Here's how the part is built. I have some questions about the finished solid (model axes, mm). Face numbers are marked on the shaded views. A direction names the side the tool comes from. Give positions to 0.01 mm unless a question says otherwise; leave off trailing zeros. Loops run counter-clockwise (first coordinate to the right, second up) from the corner with the lowest first, then second, coordinate; pieces in that order, holes last.
Q1. Suppose I cut it at B-B (z = 5). List the corners of the cut face in (x, y) for me, and give its area (3 significant figures).
Q2. Thinking about a two-plate mould opening in Z: for the marked faces 1, 2, 3 and 4, which applies, pulls with the +Z half, pulls with the -Z half, needs draft (parallel to the pull), parting line crosses it, or undercut?
Q3. Suppose I cut it at A-A (x = 4.5). List the corners of the cut face in (y, z) for me, and give its area (3 significant figures).
Q4. Suppose I cut it at C-C (x = 0). List the corners of the cut face in (y, z) for me.
Q5. Suppose I cut it at D-D (y = -2.75). List the corners of the cut face in (x, z) for me.
Q6. For the marked faces 5 and 6, which set-ups out of +Z, -Z, +X, -X, +Y, -Y let a thin tool reach every point of the face, with its end or its side?
Q7. I'm going to push a flat-ended pin straight in: P1, Ø4, axis at x = 1.5, z = 13.5, coming from the +Y side. Where does the tip first touch, or does it pass through?
Q8. I need wall thicknesses on probe 1 along Z at (x, y) = (3.25, 2); probe 2 along Y at (x, z) = (-0.25, 16.75); probe 3 along Y at (x, z) = (-2.25, 5.75). Which ranges of each line are inside material? Lowest first, please.
```python
from build123d import *

# Parameters (mm, degrees)
F1_DEPTH = 4
F2_R     = 3.5
F3_DEPTH = 12
F4_R     = 3.5
F5_DEPTH = 4


with BuildPart() as f1:
    # F0 (on Top) → F1 (new body)
    with BuildSketch(Plane.XY):
        Polygon((2.988754, -5.202629), (5.999986, -0.012978), (3.011232, 5.189651), (-2.988754, 5.202629), (-5.999986, 0.012978), (-3.011232, -5.189651), align=None)
    extrude(amount=F1_DEPTH)

    # F2 (on face) → F3 (join)
    with BuildSketch(Plane.XY.offset(4)):
        Circle(F2_R)
    extrude(amount=F3_DEPTH)

    # F4 (on face) → F5 (join)
    with BuildSketch(Plane.XY.offset(16)):
        Polygon((3.002019, -5.180605), (6.013252, 0.009046), (3.024498, 5.211675), (-2.975488, 5.224653), (-5.98672, 0.035002), (-2.997967, -5.167627), align=None)
        Circle(F4_R, mode=Mode.SUBTRACT)
        Circle(F4_R)
    extrude(amount=F5_DEPTH)


solid = f1.part
```
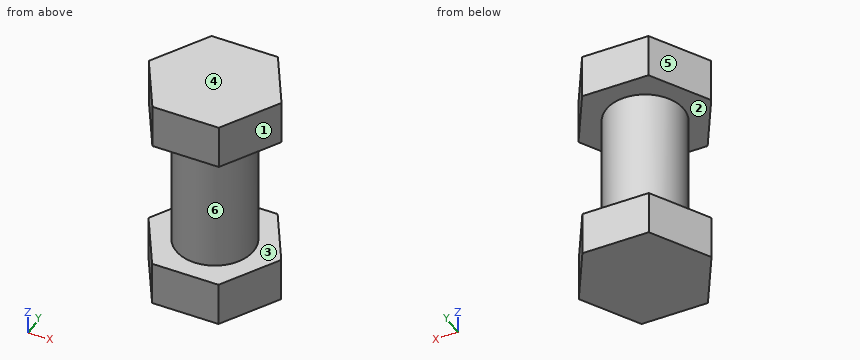
Solutions:
1. outline: circle Ø7 at (0, 0)
1. area: 38.5 mm2
2. face 1: needs draft
2. face 2: undercut
2. face 3: undercut
2. face 4: pulls with the +Z half
3. outline: (-2.6, 0) - (2.6, 0) - (2.6, 4) - (-2.6, 4) - close; (-2.6, 16) - (2.64, 16) - (2.64, 20) - (-2.6, 20) - close
3. area: 41.8 mm2
4. outline: (-5.2, 0) - (5.2, 0) - (5.2, 4) - (3.5, 4) - (3.5, 16) - (5.22, 16) - (5.22, 20) - (-5.17, 20) - (-5.17, 16) - (-3.5, 16) - (-3.5, 4) - (-5.2, 4) - close
5. outline: (-4.41, 0) - (4.41, 0) - (4.41, 4) - (2.17, 4) - (2.17, 16) - (4.41, 16) - (4.41, 20) - (-4.39, 20) - (-4.39, 16) - (-2.17, 16) - (-2.17, 4) - (-4.41, 4) - close
6. face 5: +Z, -Z, -X, +Y
6. face 6: none
7. P1: stops at y = 3.5
8. probe 1: z = 0 to 4, 16 to 20
8. probe 2: y = -5.17 to 5.22
8. probe 3: y = -2.68 to 2.68
